Solid Edge part; units mm, degrees
sketch "Sketch1" plane through (0, 0, 0) normal (0, 0, 1) x (1, 0, 0)
  circle A0 centre (0, 58) radius 1.5
  circle A1 centre (96, 58) radius 1.5
  circle A2 centre (96, 0) radius 1.5
  line L0 (-3, -3) -> (-3, 61)
  line L1 (-3, 61) -> (99, 61)
  line L2 (99, 61) -> (99, -3)
  line L3 (99, -3) -> (-3, -3)
  circle A3 centre (0, 0) radius 1.5
extrude "Protrusion1" add sketch "Sketch1" along normal blind 0.8
properties material "Epoxy, cast rigid"
CAD build for the part. Positions are in the model's coordinates, mm. Round coordinates to 2 decimals unless told otherwise and drop trailing zeros. Order: outer loops, then holes, each group sorted by start corner. A loop starts at its lowest first (then second) coordinate and runs counter-clockwise, first axis right, second up.
Item 1: Probe line 1 along Y through (x, z) = (0, 0.6). List the from-to ranges inside material, lowest first.
Item 2: Pin check, flat tip, straight feed: pin 1 (5 mm diameter, centred on x = 96, y = 58, fed in from +Z). Stop position of the tip, or through.
Item 3: Saw through at B-B on x = 96. Write the cut outline in (y, z), then the cut area to 3 significant figures.
Item 4: Mould opens along X. For faces 1 (the face through (96.806, 56.735, 0.394)), 2 (the face through (49, 29, 0)) say: pulls with the +X half, pulls with the -X half, needs draft (parallel to the pull), parting line crosses it, or undercut.
Item 5: Saw through at A-A on y = 58. Write the cut outline in (x, z).
Reported:
1. line 1: y = -3 to -1.5, 1.5 to 56.5, 59.5 to 61
2. pin 1: stops at z = 0.8
3. outline: (-3, 0) - (-1.5, 0) - (-1.5, 0.8) - (-3, 0.8) - close; (1.5, 0) - (56.5, 0) - (56.5, 0.8) - (1.5, 0.8) - close; (59.5, 0) - (61, 0) - (61, 0.8) - (59.5, 0.8) - close
3. area: 46.4 mm2
4. face 1: undercut
4. face 2: needs draft
5. outline: (-3, 0) - (-1.5, 0) - (-1.5, 0.8) - (-3, 0.8) - close; (1.5, 0) - (94.5, 0) - (94.5, 0.8) - (1.5, 0.8) - close; (97.5, 0) - (99, 0) - (99, 0.8) - (97.5, 0.8) - close
